Work out the finished part from the listing and answer in its coordinate system (mm). Face numbers are marked on the shaded views. A direction names the side the tool comes from. Round coordinates to 2 decimals unless told otherwise and drop trailing zeros. Order: outer loops, then holes, each group sorted by start corner. A loop starts at its lowest first (then second) coordinate and runs counter-clockwise, first axis right, second up. Notation, with made-up numbers: (11, 72.5) - (32, 72.5) arc R33 ccw to (32, 108.5) - close; hole circle Ø9 at (-33, 83). An arc over 180 degrees is marked (long way). Use one line per item in the form item = value. Start each with the question number.
Q1. Find the intervals of material crossed by line 1 (X direction, y = 3, z = 6.5); line 2 (X direction, y = 2.15, z = -15); line 3 (Z direction, x = 6.25, y = 0.45), in increasing order. Write a range as [from, to].
Q2. The part is cut by section A-A on x = -1.5. Determine the outline of the cut face in (y, z).
Q3. The part is cut by section C-C on z = 3. Determine the outline of the cut face in (x, y).
Q4. The part is cut by section D-D on x = 7. Determine the outline of the cut face in (y, z), plus the area to 3 significant figures.
Q5. For a pull along Z with two mould halves and no side action, classify the marked faces 3, 4 and 5 as +Z half, -Z half, draft (parallel to the pull), parting line (faces both ways), or undercut.
Q6. The part is cut by section B-B on y = 1.4. Determine the outline of the cut face in (x, z).
Q7. Which of the six approach directions +Z, -Z, +X, -X, +Y, -Y give full straight-line access (tool end or side, diameter ignored) to the marked faces 1 and 2?
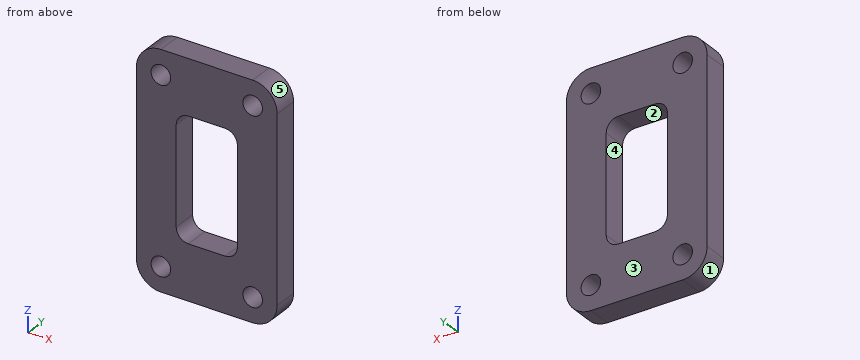
from build123d import *

# Parameters (mm, degrees)
SKETCH1_R           = 1.6
BOSS_EXTRUDE1_DEPTH = 4
CUT_EXTRUDE1_DEPTH  = 23.566568193


with BuildPart() as part:
    # Sketch1 → Boss-Extrude1 (new body)
    with BuildSketch(Plane(origin=(0, 0, 0), x_dir=(1, 0, 0), z_dir=(0, 1, 0))):
        with BuildLine():
            Line((-11.5, 15), (-11.5, -15))
            ThreePointArc((-11.5, -15), (-10.328427125, -17.828427125), (-7.5, -19))
            Line((-7.5, -19), (7.5, -19))
            ThreePointArc((7.5, -19), (10.328427125, -17.828427125), (11.5, -15))
            Line((11.5, -15), (11.5, 15))
            ThreePointArc((11.5, 15), (10.328427125, 17.828427125), (7.5, 19))
            Line((7.5, 19), (-7.5, 19))
            ThreePointArc((-7.5, 19), (-10.328427125, 17.828427125), (-11.5, 15))
        make_face()
        with Locations(Location((-7.5, 15, 0), (0, 0, 270))):
            Circle(SKETCH1_R, mode=Mode.SUBTRACT)
        with Locations(Location((7.5, 15, 0), (0, 0, 270))):
            Circle(SKETCH1_R, mode=Mode.SUBTRACT)
        with Locations(Location((-7.5, -15, 0), (0, 0, 270))):
            Circle(SKETCH1_R, mode=Mode.SUBTRACT)
        with Locations(Location((7.5, -15, 0), (0, 0, 270))):
            Circle(SKETCH1_R, mode=Mode.SUBTRACT)
    extrude(amount=BOSS_EXTRUDE1_DEPTH)

    # Sketch2 → Cut-Extrude1 (cut, through all)
    with BuildSketch(Plane(origin=(0, 4, 0), x_dir=(1, 0, 0), z_dir=(0, 1, 0))):
        with BuildLine():
            Line((-3, 10), (3, 10))
            ThreePointArc((3, 10), (4.414213562, 9.414213562), (5, 8))
            Line((5, 8), (5, -8))
            ThreePointArc((5, -8), (4.414213562, -9.414213562), (3, -10))
            Line((3, -10), (-3, -10))
            ThreePointArc((-3, -10), (-4.414213562, -9.414213562), (-5, -8))
            Line((-5, -8), (-5, 8))
            ThreePointArc((-5, 8), (-4.414213562, 9.414213562), (-3, 10))
        make_face()
    extrude(amount=-CUT_EXTRUDE1_DEPTH, mode=Mode.SUBTRACT)


solid = part.part
Found:
q1.line_1 = [-11.5, -5], [5, 11.5]
q1.line_2 = [-11.5, -9.1], [-5.9, 5.9], [9.1, 11.5]
q1.line_3 = [-19, -16], [-14, 14], [16, 19]
q2.outline = (0, -19) - (4, -19) - (4, -10) - (0, -10) - close; (0, 10) - (4, 10) - (4, 19) - (0, 19) - close
q3.outline = (-11.5, 0) - (-5, 0) - (-5, 4) - (-11.5, 4) - close; (5, 0) - (11.5, 0) - (11.5, 4) - (5, 4) - close
q4.outline = (0, -19) - (4, -19) - (4, -16.52) - (0, -16.52) - close; (0, -13.48) - (4, -13.48) - (4, 13.48) - (0, 13.48) - close; (0, 16.52) - (4, 16.52) - (4, 19) - (0, 19) - close
q4.area = 128 mm²
q5.face_3 = draft
q5.face_4 = undercut
q5.face_5 = +Z half
q6.outline = (-11.5, -15) arc R4 ccw to (-7.5, -19) - (7.5, -19) arc R4 ccw to (11.5, -15) - (11.5, 15) arc R4 ccw to (7.5, 19) - (-7.5, 19) arc R4 ccw to (-11.5, 15) - close; hole circle Ø3.2 at (-7.5, -15); hole circle Ø3.2 at (-7.5, 15); hole (-5, -8) arc R2 ccw to (-3, -10) - (3, -10) arc R2 ccw to (5, -8) - (5, 8) arc R2 ccw to (3, 10) - (-3, 10) arc R2 ccw to (-5, 8) - close; hole circle Ø3.2 at (7.5, -15); hole circle Ø3.2 at (7.5, 15)
q7.face_1 = -Z, -X, +Y, -Y
q7.face_2 = +Y, -Y
